Read the model definition and answer for the solid it produces. Units are mm, in the model's axes. Face numbers are marked on the shaded views. A direction names the side the tool comes from. Give positions to 0.01 mm unless a question says otherwise; leave off trailing zeros. Write each loop counter-clockwise with the first axis right and the second up, starting at its lowest first coordinate (ties: lowest second). Pieces come first, ordered by that corner, then holes. Notation, with made-up numbers: (-19, 26) -> (4, 26) arc R22 ccw to (4, 55) -> close; hole circle Ø5 at (83, 78). An arc over 180 degrees is marked (long way). Use a Markdown table: item, result.
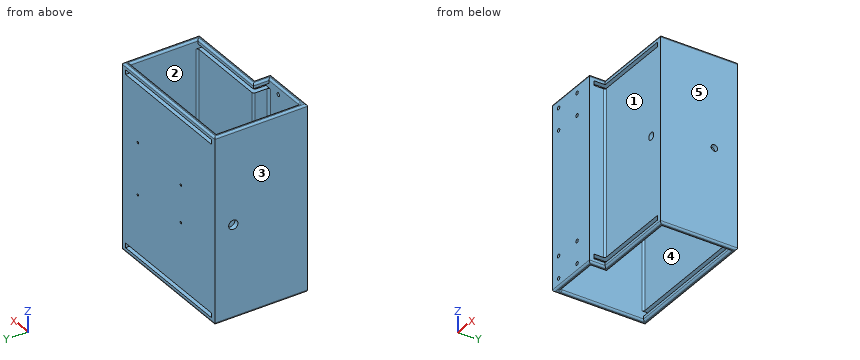
from build123d import *

# Parameters (mm, degrees)
SKETCH1_W           = 150
SKETCH1_H           = 200
BOSS_EXTRUDE1_DEPTH = 100
SHELL2_T            = -5
SKETCH5_R           = 1.9
CUT_EXTRUDE2_DEPTH  = 10
BOSS_EXTRUDE4_DEPTH = 200
SKETCH9_W           = 101.133931545
SKETCH9_H           = 31.996148617
CUT_EXTRUDE4_DEPTH  = 236.849528301
SKETCH10_R          = 4
CUT_EXTRUDE5_DEPTH  = 10
CUT_EXTRUDE7_REACH  = 162.078
SKETCH11_W          = 140
SKETCH11_H          = 5
SKETCH15_R          = 1.2
CUT_EXTRUDE11_DEPTH = 10
SKETCH36_W          = 60
SKETCH36_H          = 5
BOSS_EXTRUDE7_DEPTH = 10
FILLET1_R           = 2
SKETCH37_R          = 3.5
CUT_EXTRUDE15_DEPTH = 60
SKETCH38_R          = 5
CUT_EXTRUDE16_DEPTH = 70


with BuildPart() as part:
    # Sketch1 → Boss-Extrude1 (new body)
    with BuildSketch(Plane(origin=(0, 0, 0), x_dir=(1, 0, 0), z_dir=(0, 1, 0))):
        Rectangle(SKETCH1_W, SKETCH1_H)
    extrude(amount=BOSS_EXTRUDE1_DEPTH)

    # Shell2
    shell2_openings = [part.faces().sort_by_distance(p)[0] for p in [
        (0, 50, -100),
        (0, 50, 100),
    ]]
    offset(amount=SHELL2_T, openings=shell2_openings, kind=Kind.INTERSECTION)

    # Sketch5 → Cut-Extrude2 (cut)
    with BuildSketch(Plane.XZ):
        with Locations(Location((-65, 91, 0), (0, 0, 270))):
            Circle(SKETCH5_R)
        with Locations(Location((-35, 91, 0), (0, 0, 270))):
            Circle(SKETCH5_R)
        with Locations(Location((-65, 67, 0), (0, 0, 270))):
            Circle(SKETCH5_R)
        with Locations(Location((-35, 67, 0), (0, 0, 270))):
            Circle(SKETCH5_R)
    cut_extrude2 = extrude(amount=-CUT_EXTRUDE2_DEPTH, mode=Mode.SUBTRACT)

    # Mirror2: Cut-Extrude2 across plane
    add(cut_extrude2.mirror(Plane.XY), mode=Mode.SUBTRACT)

    # Sketch8 → Boss-Extrude4 (add, through all)
    with BuildSketch(Plane.XY.offset(100)):
        Polygon((-15, 17), (75, 17), (75, 22), (-20, 22), (-20, 0), (-15, 0), align=None)
    extrude(amount=-BOSS_EXTRUDE4_DEPTH)

    # Sketch9 → Cut-Extrude4 (cut, through all)
    with BuildSketch(Plane.XY.offset(100)):
        with Locations((35.566965773, 1.001925691)):
            Rectangle(SKETCH9_W, SKETCH9_H)
    extrude(amount=-CUT_EXTRUDE4_DEPTH, mode=Mode.SUBTRACT)

    # Sketch10 → Cut-Extrude5 (cut)
    with BuildSketch(Plane.XZ.offset(-17)):
        with Locations((60, 0)):
            Circle(SKETCH10_R)
    extrude(amount=-CUT_EXTRUDE5_DEPTH, mode=Mode.SUBTRACT)

    # Cut-Extrude7: up to this face of the body (flat: up to its plane)
    cut_extrude7_end = Plane(part.part.faces().sort_by_distance((-44.954220044, 5, 0))[0])
    # Sketch11 → Cut-Extrude7 (cut, up to the picked face)
    with BuildSketch(Plane(origin=(0, 100, 0), x_dir=(1, 0, 0), z_dir=(0, 1, 0)), mode=Mode.PRIVATE) as cut_extrude7_sk1:
        with Locations((0, -92.5)):
            Rectangle(SKETCH11_W, SKETCH11_H)
    cut_extrude7_tool1 = split(extrude(cut_extrude7_sk1.sketch, amount=-CUT_EXTRUDE7_REACH, mode=Mode.PRIVATE), bisect_by=cut_extrude7_end, keep=Keep.BOTH, mode=Mode.PRIVATE)
    cut_extrude7 = cut_extrude7_tool1.solids().sort_by(Axis((0, 100, 92.5), (0, -1, 0)))[0]
    add(cut_extrude7, mode=Mode.SUBTRACT)

    # Mirror3: Cut-Extrude7 across plane
    add(cut_extrude7.mirror(Plane.XY), mode=Mode.SUBTRACT)

    # Sketch15 → Cut-Extrude11 (cut)
    with BuildSketch(Plane(origin=(0, 100, 0), x_dir=(1, 0, 0), z_dir=(0, 1, 0))):
        with Locations(Location((50, 28, 0), (0, 0, 270))):
            Circle(SKETCH15_R)
        with Locations(Location((50, -28, 0), (0, 0, 270))):
            Circle(SKETCH15_R)
        with Locations(Location((-20, 20, 0), (0, 0, 270))):
            Circle(SKETCH15_R)
        with Locations(Location((-20, -20, 0), (0, 0, 270))):
            Circle(SKETCH15_R)
    extrude(amount=-CUT_EXTRUDE11_DEPTH, mode=Mode.SUBTRACT)

    # Sketch36 → Boss-Extrude7 (add)
    with BuildSketch(Plane.ZY.offset(-70)):
        with Locations((-13.202053215, 62.5)):
            Rectangle(SKETCH36_W, SKETCH36_H)
    boss_extrude7 = extrude(amount=BOSS_EXTRUDE7_DEPTH)

    # Mirror5: Boss-Extrude7 across plane
    add(boss_extrude7.mirror(Plane(origin=(0, 0, 0), x_dir=(0, 0, 1), z_dir=(1, 0, 0))))

    # Fillet1
    fillet1_edges = [part.edges().sort_by_distance(p)[0] for p in [
        (-45, 0, -100),
        (-20, 5, 0),
        (70, 22, 0),
        (70, 95, 0),
        (0, 100, 100),
        (70, 58.5, 100),
        (70, 58.5, -100),
        (-70, 5, 0),
        (-70, 50, -100),
        (-45, 5, 100),
        (-70, 50, 100),
        (0, 95, -100),
        (0, 95, 100),
        (-20, 22, 0),
        (-70, 95, 0),
        (-15, 17, 0),
        (70, 60, -13.202053215),
        (70, 65, -13.202053215),
        (-70, 60, -13.202053215),
        (-70, 65, -13.202053215),
        (-45, 0, 100),
        (-45, 5, -100),
        (75, 58.5, 100),
        (-75, 50, 100),
        (-75, 50, -100),
        (75, 58.5, -100),
        (-15, 8.5, 100),
        (25, 22, 100),
        (-20, 13.5, -100),
        (30, 17, -100),
        (25, 22, -100),
        (-20, 13.5, 100),
        (-15, 8.5, -100),
        (30, 17, 100),
        (0, 100, -100),
    ]]
    fillet(fillet1_edges, radius=FILLET1_R)

    # Sketch37 → Cut-Extrude15 (cut)
    with BuildSketch(Plane(origin=(75, 0, 0), x_dir=(0, 0, -1), z_dir=(1, 0, 0))):
        with Locations((0, 75)):
            Circle(SKETCH37_R)
    extrude(amount=-CUT_EXTRUDE15_DEPTH, mode=Mode.SUBTRACT)

    # Sketch38 → Cut-Extrude16 (cut)
    with BuildSketch(Plane.ZY.offset(75)):
        with Locations((0, 80)):
            Circle(SKETCH38_R)
    extrude(amount=-CUT_EXTRUDE16_DEPTH, mode=Mode.SUBTRACT)


solid = part.part
Item 1: Straight lines are drawn through the part: line 1 along Z through (x, y) = (60, 19); line 2 along X through (y, z) = (3.45, 67); line 3 along Y through (x, z) = (-58, 18.5). For each, find the intervals that lie inside material, in ascending order. Write a range as [from, to].
Return value:
| item | result |
|---|---|
| line 1 | [-100, -95], [-90, -4], [4, 90], [95, 100] |
| line 2 | [-75, -66.9], [-63.1, -36.9], [-33.1, -15] |
| line 3 | [0, 5], [95, 100] |
Item 2: A tool of negligible diameter and unlimited length cuts with its end or side. For the marked faces 4 and 5, from which of +Z, -Z, +X, -X, +Y, -Y can it reach the whole face along a straight path? Write none if from no direction.
Return value:
| item | result |
|---|---|
| face 4 | +Z, -Z |
| face 5 | +Z, -Z, +X, +Y, -Y |
Item 3: For a pull along Y with two mould halves and no side action, classify the marked faces 1, 2 and 3 as +Y half, -Y half, draft (parallel to the pull), parting line (faces both ways), or undercut.
Return value:
| item | result |
|---|---|
| face 1 | -Y half |
| face 2 | undercut |
| face 3 | draft |
Item 4: A cutting plane is placed at A-A (x = -54). Give the vertices of the cut face in (y, z).
Return value:
| item | result |
|---|---|
| outline | (0, -98) arc R2 ccw to (2, -100) -> (3, -100) arc R2 ccw to (5, -98) -> (5, 98) arc R2 ccw to (3, 100) -> (2, 100) arc R2 ccw to (0, 98) -> close; (95, -98) arc R2 ccw to (97, -100) -> (98, -100) arc R2 ccw to (100, -98) -> (100, -95) -> (95, -95) -> close; (95, -90) -> (100, -90) -> (100, 90) -> (95, 90) -> close; (95, 95) -> (100, 95) -> (100, 98) arc R2 ccw to (98, 100) -> (97, 100) arc R2 ccw to (95, 98) -> close |
Item 5: A cutting plane is placed at D-D (y = 53.5). Give the vertices of the cut face in (x, z).
Return value:
| item | result |
|---|---|
| outline | (-75, -98) arc R2 ccw to (-73, -100) -> (-72, -100) arc R2 ccw to (-70, -98) -> (-70, 98) arc R2 ccw to (-72, 100) -> (-73, 100) arc R2 ccw to (-75, 98) -> close; (70, -98) arc R2 ccw to (72, -100) -> (73, -100) arc R2 ccw to (75, -98) -> (75, 98) arc R2 ccw to (73, 100) -> (72, 100) arc R2 ccw to (70, 98) -> close |
Item 6: Each of these flat-tipped pins is pushed along its axis until it touches: P1, Ø2, axis at x = 40, z = -27.5, coming from the -Y side; P2, Ø13.5, axis at y = 7.5, z = -29.5, coming from the +X side; P3, Ø10, axis at x = 62.5, y = 60.5, coming from the +Z side. Where does it stop, or does it pass through?
Return value:
| item | result |
|---|---|
| P1 | y = 17 |
| P2 | x = -15 |
| P3 | z = 16.8 |
Item 7: A cutting plane is placed at B-B (y = 10). Give the vertices of the cut face in (x, z), then the cut area to 3 significant figures.
Return value:
| item | result |
|---|---|
| outline | (-75, -98) arc R2 ccw to (-73, -100) -> (-72, -100) arc R2 ccw to (-70, -98) -> (-70, 98) arc R2 ccw to (-72, 100) -> (-73, 100) arc R2 ccw to (-75, 98) -> close; (-20, -98) arc R2 ccw to (-18, -100) -> (-17, -100) arc R2 ccw to (-15, -98) -> (-15, -95) -> (-20, -95) -> close; (-20, -90) -> (-15, -90) -> (-15, 90) -> (-20, 90) -> close; (-20, 95) -> (-15, 95) -> (-15, 98) arc R2 ccw to (-17, 100) -> (-18, 100) arc R2 ccw to (-20, 98) -> close |
| area | 1,940 mm^2 |
Item 8: A cutting plane is placed at C-C (z = 74.5). Give the vertices of the cut face in (x, y), then the cut area to 3 significant figures.
Return value:
| item | result |
|---|---|
| outline | (-75, 0) -> (-15, 0) -> (-15, 15) arc R2 cw to (-13, 17) -> (75, 17) -> (75, 100) -> (-75, 100) -> close; hole (-70, 7) arc R2 ccw to (-68, 5) -> (-22, 5) arc R2 ccw to (-20, 7) -> (-20, 20) arc R2 cw to (-18, 22) -> (68, 22) arc R2 ccw to (70, 24) -> (70, 93) arc R2 ccw to (68, 95) -> (-68, 95) arc R2 ccw to (-70, 93) -> close |
| area | 2,400 mm^2 |
